```python
from build123d import *

# Parameters (mm, degrees)
SKETCH1_R           = 6.35
BOSS_EXTRUDE1_DEPTH = 19.05
SKETCH2_R           = 12.7
CUT_EXTRUDE1_DEPTH  = 12.7


with BuildPart() as part:
    # Sketch1 → Boss-Extrude1 (new body)
    with BuildSketch(Plane.XY):
        with BuildLine():
            Line((568.345160721, 503.256723569), (304.695644733, 282.028511943))
            ThreePointArc((304.695644733, 282.028511943), (301.564919628, 246.244179632), (337.349251645, 243.113451162))
            Line((337.349251645, 243.113451162), (600.998771294, 464.341665859))
            ThreePointArc((600.998771294, 464.341665859), (604.129494863, 500.126), (568.345160721, 503.256723569))
        make_face()
        with Locations(Location((321.022448189, 262.570981553, 0), (0, 0, 180))):
            Circle(SKETCH1_R, mode=Mode.SUBTRACT)
        with Locations(Location((584.671966007, 483.799194714, 0), (0, 0, 180))):
            Circle(SKETCH1_R, mode=Mode.SUBTRACT)
        with BuildLine():
            Line((563.649075368, 449.580222357), (358.372145945, 277.33242659))
            ThreePointArc((358.372145945, 277.33242659), (340.479978874, 278.897788374), (342.045340659, 296.789955445))
            Line((342.045340659, 296.789955445), (547.322270082, 469.037751213))
            ThreePointArc((547.322270082, 469.037751213), (565.214437152, 467.472389428), (563.649075368, 449.580222357))
        make_face(mode=Mode.SUBTRACT)
    extrude(amount=BOSS_EXTRUDE1_DEPTH)

    # Sketch2 → Cut-Extrude1 (cut)
    with BuildSketch(Plane.XY.offset(19.05)):
        with Locations((321.022448189, 262.570981553)):
            Circle(SKETCH2_R)
        with Locations((584.671966007, 483.799194714)):
            Circle(SKETCH2_R)
    extrude(amount=-CUT_EXTRUDE1_DEPTH, mode=Mode.SUBTRACT)


solid = part.part
```
Geometry check sheet. Reference: the model listing, model coordinates, mm. A direction names the side the tool comes from. Give positions to 0.01 mm unless a question says otherwise; leave off trailing zeros. Write each loop counter-clockwise with the first axis right and the second up, starting at its lowest first coordinate (ties: lowest second). Pieces come first, ordered by that corner, then holes.
1) Section check A-A, the plane x = 347.5. Record the boundary of the cut face in (y, z), and give its area (3 significant figures).
2) Section check B-B, the plane y = 456.5. Record the boundary of the cut face in (x, z), and give its area (3 significant figures).
3) Release check for a two-part mould opening along Y. For faces 4 (the flat face through (462.448, 364.662, 9.392)), 5 (the cylindrical face through (301.211, 246.676, 9.392)), 6 (the flat face through (438.366, 394.191, 9.392)), 7 (the cylindrical face through (340.66, 278.69, 9.39)) record: pulls with the +Y half, pulls with the -Y half, needs draft (parallel to the pull), parting line crosses it, or undercut.
4) Gauge pin test, flat ends, axial feed: pin 1 (16.5 mm diameter, centred on x = 321.02, y = 262.57, fed in from +Z); pin 2 (4 mm diameter, centred on y = 441.5, z = 10.5, fed in from +X); pin 3 (6 mm diameter, centred on y = 457, z = 15.5, fed in from +X). Record the tip position at first contact, or that the pin passes through.
5) Access from +Z, -Z, +X, -X, +Y, -Y to the whole of each face (thin tool, end or side, straight path). Record for faces 1 (the flat face through (467.33, 352.18, 9.39)), 2 (the flat face through (443.25, 381.71, 9.39)), 3 (the cylindrical face through (575.31, 492.38, 12.79)).
6) Section check C-C, the plane z = 9.5. Record the boundary of the cut face in (x, y).
7) Material ranges on L1, parallel to X at y = 332, z = 6; L2, parallel to Y at x = 498.5, z = 2; L3, parallel to X at y = 405, z = 4.75, recorded low to high.
Computed:
1. outline: (251.63, 0) - (274.65, 0) - (274.65, 19.05) - (251.63, 19.05) - close; (301.37, 0) - (317.95, 0) - (317.95, 19.05) - (301.37, 19.05) - close
1. area: 754 mm2
2. outline: (512.62, 0) - (532.38, 0) - (532.38, 19.05) - (512.62, 19.05) - close; (567.87, 0) - (591.65, 0) - (591.65, 19.05) - (567.87, 19.05) - close
2. area: 829 mm2
3. face 4: undercut
3. face 5: parting line crosses it
3. face 6: pulls with the +Y half
3. face 7: undercut
4. pin 1: stops at z = 6.35
4. pin 2: stops at x = 576.16
4. pin 3: stops at x = 595.82
5. face 1: +Z, -Z, +X, -Y
5. face 2: +Z, -Z
5. face 3: +Z
6. outline: (304.7, 282.03) arc R25.4 ccw to (337.35, 243.11) - (601, 464.34) arc R25.4 ccw to (568.35, 503.26) - close; hole circle Ø25.4 at (321.02, 262.57); hole (342.05, 296.79) arc R12.7 ccw to (358.37, 277.33) - (563.65, 449.58) arc R12.7 ccw to (547.32, 469.04) - close; hole circle Ø25.4 at (584.67, 483.8)
7. L1: x = 364.25 to 384.01, 423.52 to 443.28
7. L2: y = 378.33 to 394.91, 428.07 to 444.65
7. L3: x = 451.25 to 471.01, 510.52 to 530.28
